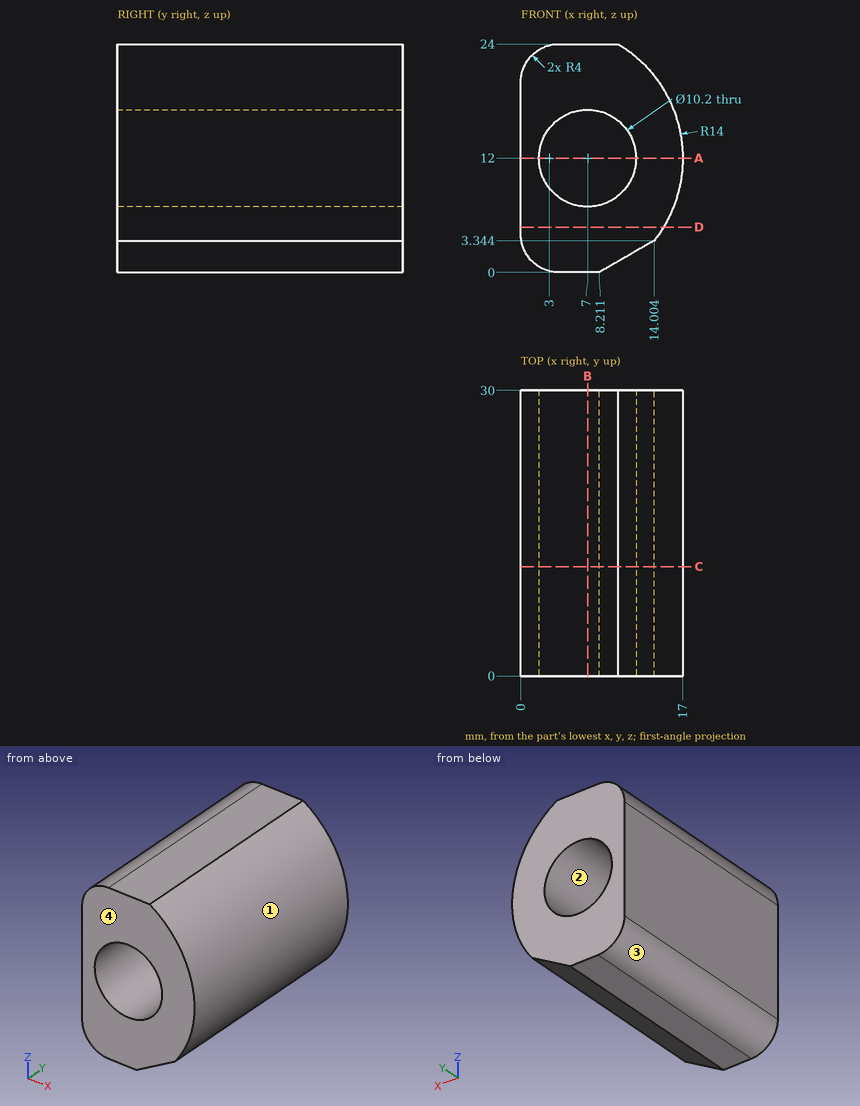
Drawing for the job (mm, zero at the part's lowest x, y, z). Give positions to 0.01 mm unless a question says otherwise; leave off trailing zeros. Loops run counter-clockwise (first coordinate to the right, second up) from the corner with the lowest first, then second, coordinate; pieces in that order, holes last. Notation, with made-up numbers: (-2.5, 74) - (5.5, 74) arc R29 cw to (5.5, 102) - close; hole circle Ø11 at (-12.75, -17.75). An arc over 180 degrees is marked (long way). Write item = value, one per line. Start each with the question number.
1) Band-saw the part on D-D on z = 4.75. Give the cut face in (x, y), plus the area to 3 significant figures.
2) Pull direction Z, two halves, no side cores. Call the marked faces 1, 2, 3 and 4: +Z half, -Z half, draft (parallel to the pull), parting line (faces both ways), or undercut.
3) Probe probe 1 along X at (y, z) = (21, 12); probe 2 along X at (y, z) = (25.75, 10.5) (1 decimal); probe 3 along Z at (x, y) = (2.5, 27.75) (1 decimal). List the from-to ranges inside material, lowest first. Write a range as from..to.
4) Band-saw the part on C-C on y = 11.5. Give the cut face in (x, z) (1 decimal), plus the area to 3 significant figures.
5) Drop flat-ended pins along their axis: pin 1 Ø3 at (x, y) = (15, 24) entering from +Z; pin 2 Ø8 at (y, z) = (14.5, 3) entering from +X; pin 3 Ø1.5 at (y, z) = (6.5, 16) entering from +X. Give the stop position or say it passes through.
6) Band-saw the part on B-B on x = 7. Give the cut face in (y, z), plus the area to 3 significant figures.
7) Band-saw the part on A-A on z = 12. Give the cut face in (x, y).
Final values:
q1.outline = (0, 0) - (14.98, 0) - (14.98, 30) - (0, 30) - close
q1.area = 449 mm²
q2.face_1 = parting line
q2.face_2 = undercut
q2.face_3 = -Z half
q2.face_4 = draft
q3.probe_1 = 0..1.9, 12.1..17
q3.probe_2 = 0..2.1, 11.9..16.9
q3.probe_3 = 0.3..9.6, 14.4..23.7
q4.outline = (0, 4) arc R4 ccw to (4, 0) - (8.2, 0) - (14, 3.3) arc R14 ccw to (10.2, 24) - (4, 24) arc R4 ccw to (0, 20) - close; hole circle Ø10.2 at (7, 12)
q4.area = 268 mm²
q5.pin_1 = 21.26
q5.pin_2 = 16.08
q5.pin_3 = 16.62
q6.outline = (0, 0) - (30, 0) - (30, 6.9) - (0, 6.9) - close; (0, 17.1) - (30, 17.1) - (30, 24) - (0, 24) - close
q6.area = 414 mm²
q7.outline = (0, 0) - (1.9, 0) - (1.9, 30) - (0, 30) - close; (12.1, 0) - (17, 0) - (17, 30) - (12.1, 30) - close
